Can you work these out from the drawing? Everything is in mm from the part's minimum corner. A direction names the side the tool comes from. Coordinates: 2 decimals unless noted, no trailing zeros. Order: outer loops, then holes, each group sorted by start corner. A loop starts at its lowest first (then second) coordinate and runs counter-clockwise, first axis right, second up. Notation, with made-up numbers: (33, 5.25) - (74, 5.25) arc R16 cw to (74, 17.25) - close; hole circle Ø10 at (88, -10). An arc over 180 degrees is marked (long way). Use a Markdown table: item, result. Add a question column.
(1) I want a section at B-B (z = 8.75). List the corners of the cut face in (x, y) for me.
(2) I want a section at D-D (y = 10.5). List the corners of the cut face in (x, z) for me, and give its area (3 significant figures).
(3) We'd pull the mould along X, two halves only. Please class the marked faces 6, 7, 8 and 9: pulls with the +X half, pulls with the -X half, needs draft (parallel to the pull), parting line crosses it, or undercut.
(4) If I drill on L1, parallel to X at y = 9.5, z = 13.25; L2, parallel to Y at x = 5.08, z = 13.85; L3, parallel to X at y = 1.75, z = 6, over which ranges is the centre line in solid material (lowest first)? Write a range as [from, to].
(5) For pin 1 Ø2.5 at (x, y) = (35.56, 9.525) entering from -Z; pin 2 Ø6 at (y, z) = (13, 8) entering from -X; pin 3 Ø11 at (x, y) = (4.5, 7) entering from -Z; pin 4 Ø6 at (y, z) = (7.5, 4.5) entering from +X, each with a flat end and sliding along its axis, tell me the tip position at first contact or that it passes through.
(6) I want a section at C-C (y = 2.5). List the corners of the cut face in (x, z) for me.
(7) On a 3-axis mill with a long thin cutter (end or side, diameter ignored), from which of +Z, -Z, +X, -X, +Y, -Y can I reach the whole of each face in a straight line? I mean the marked faces 1, 2, 3, 4 and 5. Say none if no direction works.
(8) I want a section at A-A (x = 35.56). List the corners of the cut face in (y, z) for me.
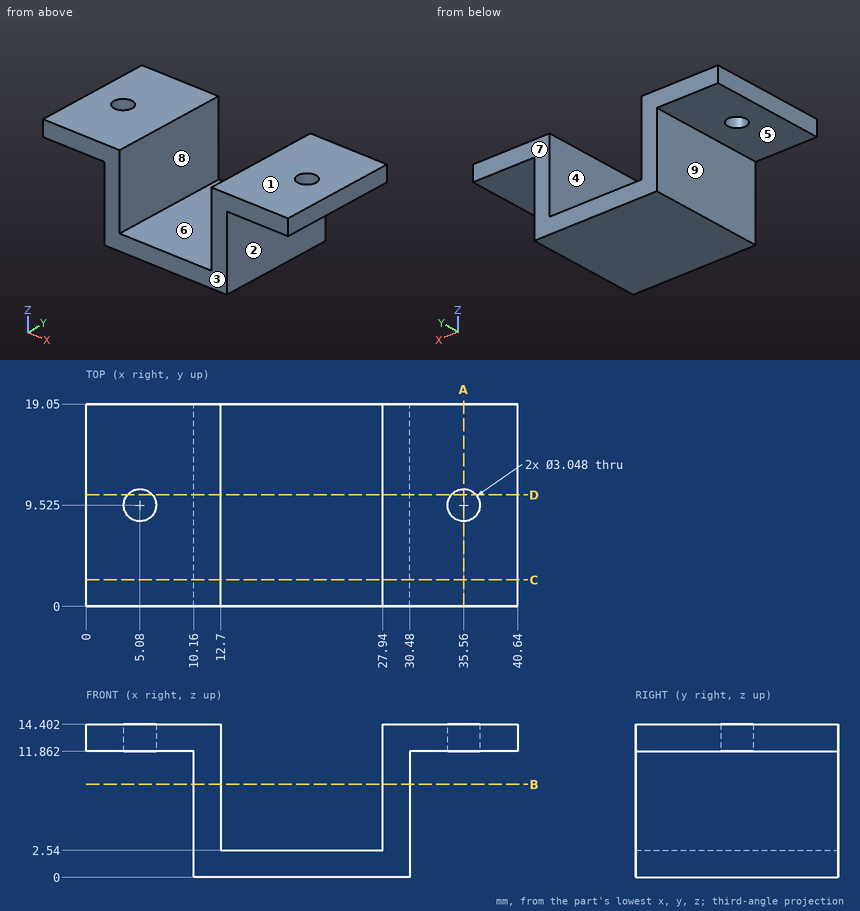
Answers follow:
| question | item | result |
|---|---|---|
| 1 | outline | (10.16, 0) - (12.7, 0) - (12.7, 19.05) - (10.16, 19.05) - close; (27.94, 0) - (30.48, 0) - (30.48, 19.05) - (27.94, 19.05) - close |
| 2 | outline | (0, 11.86) - (3.91, 11.86) - (3.91, 14.4) - (0, 14.4) - close; (6.25, 11.86) - (10.16, 11.86) - (10.16, 0) - (30.48, 0) - (30.48, 11.86) - (34.39, 11.86) - (34.39, 14.4) - (27.94, 14.4) - (27.94, 2.54) - (12.7, 2.54) - (12.7, 14.4) - (6.25, 14.4) - close; (36.73, 11.86) - (40.64, 11.86) - (40.64, 14.4) - (36.73, 14.4) - close |
| 2 | area | 152 mm² |
| 3 | face 6 | undercut |
| 3 | face 7 | needs draft |
| 3 | face 8 | undercut |
| 3 | face 9 | pulls with the -X half |
| 4 | L1 | x = [0, 3.56], [6.6, 12.7], [27.94, 34.04], [37.08, 40.64] |
| 4 | L2 | y = [0, 8], [11.05, 19.05] |
| 4 | L3 | x = [10.16, 12.7], [27.94, 30.48] |
| 5 | pin 1 | passes through |
| 5 | pin 2 | stops at x = 10.16 |
| 5 | pin 3 | stops at z = 11.86 |
| 5 | pin 4 | stops at x = 30.48 |
| 6 | outline | (0, 11.86) - (10.16, 11.86) - (10.16, 0) - (30.48, 0) - (30.48, 11.86) - (40.64, 11.86) - (40.64, 14.4) - (27.94, 14.4) - (27.94, 2.54) - (12.7, 2.54) - (12.7, 14.4) - (0, 14.4) - close |
| 7 | face 1 | +Z, +X, -X, +Y, -Y |
| 7 | face 2 | -Z, +X, +Y, -Y |
| 7 | face 3 | +Z, -Z, +X, -X, -Y |
| 7 | face 4 | +Z, +Y, -Y |
| 7 | face 5 | -Z, -X, +Y, -Y |
| 8 | outline | (0, 11.86) - (8, 11.86) - (8, 14.4) - (0, 14.4) - close; (11.05, 11.86) - (19.05, 11.86) - (19.05, 14.4) - (11.05, 14.4) - close |
